Read the model definition and answer for the solid it produces. Units are mm, in the model's axes. Face numbers are marked on the shaded views. A direction names the side the tool comes from. Give positions to 0.01 mm unless a question says otherwise; leave off trailing zeros. Loops run counter-clockwise (first coordinate to the right, second up) from the corner with the lowest first, then second, coordinate; pieces in that order, holes last. Notation, with made-up numbers: (-13.5, -23) -> (6.5, -23) arc R27 cw to (6.5, 7) -> close; hole circle Ø8 at (-7, 8). An arc over 180 degrees is marked (long way). One line per item, written item: value. Start each with the question number.
from build123d import *

# Parameters (mm, degrees)
SKETCH1_R           = 40
BOSS_EXTRUDE1_DEPTH = 10
SKETCH3_R           = 40
SKETCH3_W           = 30
SKETCH3_H           = 46.499999994
BOSS_EXTRUDE3_DEPTH = 25
CUT_EXTRUDE1_START  = -35
CUT_EXTRUDE1_DEPTH  = 35
SKETCH5_R           = 2.55
CUT_EXTRUDE2_DEPTH  = 5
CUT_EXTRUDE3_DEPTH  = 25
CUT_EXTRUDE4_DEPTH  = 22
SKETCH9_R           = 1
CUT_EXTRUDE5_DEPTH  = 10
SKETCH10_R          = 1.299999998
SKETCH10_R_2        = 1.299999999
SKETCH10_R_3        = 1.3
CUT_EXTRUDE6_DEPTH  = 10
CHAMFER1_SIZE       = 5


with BuildPart() as part:
    # Sketch1 → Boss-Extrude1 (new body)
    with BuildSketch(Plane.XY):
        with Locations((0, 222.499999997)):
            Circle(SKETCH1_R)
    extrude(amount=BOSS_EXTRUDE1_DEPTH)

    # Sketch3 → Boss-Extrude3 (add)
    with BuildSketch(Plane.XY.offset(10)):
        with Locations((0, 222.499999997)):
            Circle(SKETCH3_R)
        with Locations((0, 222.499999997)):
            Rectangle(SKETCH3_W, SKETCH3_H, mode=Mode.SUBTRACT)
    extrude(amount=BOSS_EXTRUDE3_DEPTH)

    # Sketch4 → Cut-Extrude1 (cut)
    with BuildSketch(Plane.XY.offset(35).offset(CUT_EXTRUDE1_START)):
        with BuildLine():
            ThreePointArc((40, 222.499999997), (38.912456167, 231.763949212), (35.708962247, 240.524150885))
            ThreePointArc((35.708962247, 240.524150885), (31.77566454, 233.14486234), (30.74061322, 224.84706751))
            ThreePointArc((30.74061322, 224.84706751), (30.809531665, 222.499999997), (30.74061322, 220.152932484))
            ThreePointArc((30.74061322, 220.152932484), (31.77566454, 211.855137653), (35.708962247, 204.475849108))
            ThreePointArc((35.708962247, 204.475849108), (38.912456167, 213.236050782), (40, 222.499999997))
        make_face()
        with BuildLine():
            ThreePointArc((-2.347067513, 191.759386777), (-10.644862344, 190.724335457), (-18.024150889, 186.79103775))
            ThreePointArc((-18.024150889, 186.79103775), (0, 182.499999997), (18.024150889, 186.79103775))
            ThreePointArc((18.024150889, 186.79103775), (10.644862344, 190.724335457), (2.347067513, 191.759386777))
            ThreePointArc((2.347067513, 191.759386777), (0, 191.690468331), (-2.347067513, 191.759386777))
        make_face()
        with BuildLine():
            ThreePointArc((18.024150889, 258.208962244), (0, 262.499999997), (-18.024150889, 258.208962244))
            ThreePointArc((-18.024150889, 258.208962244), (-10.644862344, 254.275664537), (-2.347067513, 253.240613217))
            ThreePointArc((-2.347067513, 253.240613217), (0, 253.309531662), (2.347067513, 253.240613217))
            ThreePointArc((2.347067513, 253.240613217), (10.644862344, 254.275664537), (18.024150889, 258.208962244))
        make_face()
        with BuildLine():
            ThreePointArc((-30.74061322, 220.152932484), (-30.809531665, 222.499999997), (-30.74061322, 224.84706751))
            ThreePointArc((-30.74061322, 224.84706751), (-31.77566454, 233.14486234), (-35.708962247, 240.524150885))
            ThreePointArc((-35.708962247, 240.524150885), (-40, 222.499999997), (-35.708962247, 204.475849108))
            ThreePointArc((-35.708962247, 204.475849108), (-31.77566454, 211.855137653), (-30.74061322, 220.152932484))
        make_face()
    extrude(amount=CUT_EXTRUDE1_DEPTH, mode=Mode.SUBTRACT)

    # Sketch5 → Cut-Extrude2 (cut)
    with BuildSketch(Plane.XY.offset(35)):
        with Locations((-22.627416998, 245.127416995)):
            Circle(SKETCH5_R)
        with Locations(Location((22.627416998, 245.127416995, 0), (0, 0, 180))):
            Circle(SKETCH5_R)
        with Locations((22.627416998, 199.872582999)):
            Circle(SKETCH5_R)
        with Locations(Location((-22.627416998, 199.872582999, 0), (0, 0, 180))):
            Circle(SKETCH5_R)
    extrude(amount=-CUT_EXTRUDE2_DEPTH, mode=Mode.SUBTRACT)

    # Sketch6 → Cut-Extrude3 (cut)
    with BuildSketch(Plane.XY.offset(35)):
        with BuildLine():
            Line((-15, 218.499999997), (-15, 226.499999997))
            ThreePointArc((-15, 226.499999997), (-19, 222.499999997), (-15, 218.499999997))
        make_face()
        with BuildLine():
            Line((15, 218.499999997), (15, 226.499999997))
            ThreePointArc((15, 226.499999997), (19, 222.499999997), (15, 218.499999997))
        make_face()
    extrude(amount=-CUT_EXTRUDE3_DEPTH, mode=Mode.SUBTRACT)

    # Sketch8 → Cut-Extrude4 (cut)
    with BuildSketch(Plane(origin=(-15, 0, 0), x_dir=(0, 0, -1), z_dir=(1, 0, 0))):
        Polygon((-22, 226.499999997), (-35, 226.499999997), (-35, 218.499999997), (-22, 218.499999997), (0, 218.499999997), (0, 226.499999997), align=None)
    extrude(amount=-CUT_EXTRUDE4_DEPTH, mode=Mode.SUBTRACT)

    # Sketch9 → Cut-Extrude5 (cut)
    with BuildSketch(Plane(origin=(0, 0, 0), x_dir=(-1, 0, 0), z_dir=(0, 0, -1))):
        with Locations((0, 222.499999997)):
            Circle(SKETCH9_R)
    extrude(amount=-CUT_EXTRUDE5_DEPTH, mode=Mode.SUBTRACT)

    # Sketch10 → Cut-Extrude6 (cut)
    with BuildSketch(Plane(origin=(0, 0, 0), x_dir=(-1, 0, 0), z_dir=(0, 0, -1))):
        with Locations((-6, 234.5)):
            Circle(SKETCH10_R)
        with Locations((6, 234.5)):
            Circle(SKETCH10_R_2)
        with Locations((6, 210.499999997)):
            Circle(SKETCH10_R_3)
        with Locations((-6, 210.499999997)):
            Circle(SKETCH10_R_3)
    extrude(amount=-CUT_EXTRUDE6_DEPTH, mode=Mode.SUBTRACT)

    # Chamfer1
    chamfer1_edges = [part.edges().sort_by_distance(p)[0] for p in [
        (-22.851493975, 218.499999997, 35),
        (-22.851493975, 226.499999997, 35),
    ]]
    chamfer(chamfer1_edges, length=CHAMFER1_SIZE)


solid = part.part
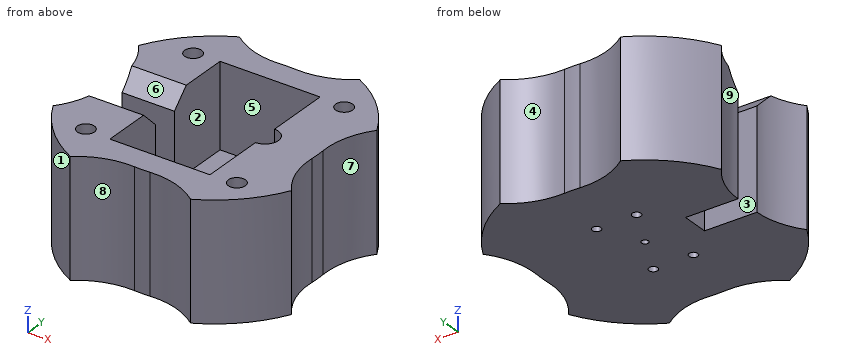
Item 1: For the marked faces 5, 6, 7, 8 and 9, determine the directions among +Z, -Z, +X, -X, +Y, -Y from which every point of the face is accessible in a straight line to the end or side of a thin tool.
Item 2: Section D-D, the plane z = 24.5 is taken. Determine the outline of the cut face in (x, y), plus the area to 3 significant figures.
Item 3: Section A-A, the plane x = 0 is taken. Determine the outline of the cut face in (y, z).
Item 4: Section C-C, the plane y = 210.5 is taken. Determine the outline of the cut face in (x, z).
Item 5: Determine the mould class of the marked faces 1, 2, 3 and 4 for opening direction X: pulls with the +X half, pulls with the -X half, needs draft (parallel to the pull), parting line crosses it, or undercut.
Item 6: Section B-B, the plane z = 3 is taken. Determine the outline of the cut face in (x, y), plus the area to 3 significant figures.
Item 7: Flat-ended cylindrical pins translate along their axes: pin 1 (1 mm diameter, centred on x = 5.5, z = 17, fed in from +Y); pin 2 (1 mm diameter, centred on x = -20, y = 217.5, fed in from +Z); pin 3 (4 mm diameter, centred on x = -7, y = 236, fed in from +Z). Find the tip coordinate at first contact, or state that the pin passes through.
Item 8: Consider L1, parallel to Y at x = -6, z = 7.25; L2, parallel to X at y = 222.5, z = 5; L3, parallel to X at y = 234.5, z = 8.25. Determine where each line is inside the solid, lowest interval first. Write a range as [from, to].
Computed values:
1. face 5: +Z
1. face 6: +Z, -X
1. face 7: +Z, -Z, +X
1. face 8: +Z, -Z, -Y
1. face 9: +Z, -Z, -X
2. outline: (-35.71, 204.48) arc R40 ccw to (-18.02, 186.79) arc R23 cw to (-2.35, 191.76) arc R40 ccw to (2.35, 191.76) arc R23 cw to (18.02, 186.79) arc R40 ccw to (35.71, 204.48) arc R23 cw to (30.74, 220.15) arc R40 ccw to (30.74, 224.85) arc R23 cw to (35.71, 240.52) arc R40 ccw to (18.02, 258.21) arc R23 cw to (2.35, 253.24) arc R40 ccw to (-2.35, 253.24) arc R23 cw to (-18.02, 258.21) arc R40 ccw to (-35.71, 240.52) arc R23 cw to (-30.7, 226.5) -> (-15, 226.5) -> (-15, 245.75) -> (15, 245.75) -> (15, 226.5) arc R4 cw to (15, 218.5) -> (15, 199.25) -> (-15, 199.25) -> (-15, 218.5) -> (-30.7, 218.5) arc R23 cw to start
2. area: 2,530 mm²
3. outline: (191.69, 0) -> (221.5, 0) -> (221.5, 10) -> (199.25, 10) -> (199.25, 35) -> (191.69, 35) -> close; (223.5, 0) -> (253.31, 0) -> (253.31, 35) -> (245.75, 35) -> (245.75, 10) -> (223.5, 10) -> close
4. outline: (-32.25, 0) -> (-7.3, 0) -> (-7.3, 10) -> (-15, 10) -> (-15, 35) -> (-32.25, 35) -> close; (-4.7, 0) -> (4.7, 0) -> (4.7, 10) -> (-4.7, 10) -> close; (7.3, 0) -> (32.25, 0) -> (32.25, 35) -> (15, 35) -> (15, 10) -> (7.3, 10) -> close
5. face 1: pulls with the -X half
5. face 2: undercut
5. face 3: needs draft
5. face 4: undercut
6. outline: (-35.71, 204.48) arc R40 ccw to (-18.02, 186.79) arc R23 cw to (-2.35, 191.76) arc R40 ccw to (2.35, 191.76) arc R23 cw to (18.02, 186.79) arc R40 ccw to (35.71, 204.48) arc R23 cw to (30.74, 220.15) arc R40 ccw to (30.74, 224.85) arc R23 cw to (35.71, 240.52) arc R40 ccw to (18.02, 258.21) arc R23 cw to (2.35, 253.24) arc R40 ccw to (-2.35, 253.24) arc R23 cw to (-18.02, 258.21) arc R40 ccw to (-35.71, 240.52) arc R23 cw to (-30.7, 226.5) -> (-15, 226.5) -> (-15, 218.5) -> (-30.7, 218.5) arc R23 cw to start; hole circle Ø2.6 at (-6, 210.5); hole circle Ø2.6 at (-6, 234.5); hole circle Ø2 at (0, 222.5); hole circle Ø2.6 at (6, 210.5); hole circle Ø2.6 at (6, 234.5)
6. area: 3,920 mm²
7. pin 1: y = 253.32
7. pin 2: z = 31.5
7. pin 3: z = 10
8. L1: [191.68, 209.2], [211.8, 233.2], [235.8, 253.32]
8. L2: [-15, -1], [1, 30.81]
8. L3: [-32.25, -7.3], [-4.7, 4.7], [7.3, 32.25]
